CAD build for the part. Positions are in the model's coordinates, mm. A direction names the side the tool comes from. Give positions to 0.01 mm unless a question says otherwise; leave off trailing zeros. Loops run counter-clockwise (first coordinate to the right, second up) from the corner with the lowest first, then second, coordinate; pieces in that order, holes last. Notation, with made-up numbers: (-33, -26.5) - (7, -26.5) arc R27 ccw to (7, 8.5) - close; hole circle Ø10 at (49.5, 11.25). An arc over 180 degrees is marked (long way). Return JSON: item names as keys, results as strings.
from build123d import *

# Parameters (mm, degrees)
F0_W           = 19
F0_H           = 55
F1_DEPTH       = 19
F3_D           = 4.4
F3_DEPTH       = 10
F3_CSINK_D     = 6
F3_CSINK_ANGLE = 90
F3_TIP         = 1.3218933619
F5_D           = 6.6
F5_DEPTH       = 10
F5_CSINK_D     = 7
F5_CSINK_ANGLE = 90
F5_TIP         = 1.9828400428


with BuildPart() as f1:
    # F0 (on Front) → F1 (new body)
    with BuildSketch(Plane.XZ):
        with Locations((9.5, -27.5)):
            Rectangle(F0_W, F0_H)
    extrude(amount=F1_DEPTH)

    # F3
    with Locations(Plane.XZ.offset(19)):
        with Locations((9.5, -7.5), (9.5, -47.5)):
            CounterSinkHole(F3_D / 2, F3_CSINK_D / 2, depth=F3_DEPTH, counter_sink_angle=F3_CSINK_ANGLE)
            with Locations((0, 0, -(F3_DEPTH + F3_TIP / 2))):  # 118° drill point
                Cone(0, F3_D / 2, F3_TIP, mode=Mode.SUBTRACT)

    # F5
    with Locations(Plane(origin=(0, 0, 0), x_dir=(-1, 0, 0), z_dir=(0, 1, 0))):
        with Locations((-9.5, -15), (-9.5, -40)):
            CounterSinkHole(F5_D / 2, F5_CSINK_D / 2, depth=F5_DEPTH, counter_sink_angle=F5_CSINK_ANGLE)
            with Locations((0, 0, -(F5_DEPTH + F5_TIP / 2))):  # 118° drill point
                Cone(0, F5_D / 2, F5_TIP, mode=Mode.SUBTRACT)


solid = f1.part
1. Drill centre lines: probe 1 along Z at (x, y) = (9.5, -3); probe 2 along Z at (x, y) = (9.5, -16); probe 3 along X at (y, z) = (-6.5, -40). Where is each one in solid material? Low to high.
Values follow:
{"probe 1": "z = -55 to -43.3, -36.7 to -18.3, -11.7 to 0", "probe 2": "z = -55 to -49.7, -45.3 to -9.7, -5.3 to 0", "probe 3": "x = 0 to 6.2, 12.8 to 19"}
2. Cut at A-A, the plane y = -4.25. Write the cut outline in (x, z).
Values follow:
{"outline": "(0, -55) - (19, -55) - (19, 0) - (0, 0) - close; hole circle Ø6.6 at (9.5, -40); hole circle Ø6.6 at (9.5, -15)"}
3. Which spindle directions (+Z, -Z, +X, -X, +Y, -Y) get a long thin tool onto all of the face, cutting with end or side? Do faces 5 (the face through (9.79, -13.54, -5.32)), 6 (the face through (7.07, -5.17, -37.77)), 7 (the face through (9, -19, -27)). Say none if no direction does.
Values follow:
{"face 5": "-Y", "face 6": "+Y", "face 7": "+Z, -Z, +X, -X, -Y"}
4. Pull direction Z, two halves, no side cores. Call faces 1 (the face through (9, -9, 0)), 2 (the face through (9.977, -13.536, -49.648)), 3 (the face through (9.71, -7.91, -47.18)), 4 (the face through (9, 0, -27)): +Z half, -Z half, draft (parallel to the pull), parting line (faces both ways), or undercut.
Values follow:
{"face 1": "+Z half", "face 2": "undercut", "face 3": "undercut", "face 4": "draft"}
5. Cut at B-B, the plane y = -11.25. Write the cut outline in (x, z).
Values follow:
{"outline": "(0, -55) - (19, -55) - (19, 0) - (0, 0) - close; hole circle Ø4.4 at (9.5, -47.5); hole circle Ø4.4 at (9.5, -7.5); hole circle Ø2.44 at (9.5, -40); hole circle Ø2.44 at (9.5, -15)"}
